Check sheet for the modelled part. Datum: model origin and axes. Units: mm. Face numbers are marked on the shaded views. A direction names the side the tool comes from. Coordinates: 2 decimals unless noted, no trailing zeros.
1. Set-up check for the marked faces 4, 5 and 6: record each of +Z, -Z, +X, -X, +Y, -Y from which the full face is reachable in a straight line by a thin tool's end or side.
2. Gauge pin test, flat ends, axial feed: pin 1 Ø1 at (x, y) = (-130.5, 9.5) entering from +Z; pin 2 Ø10.5 at (x, z) = (-103.5, 16) entering from +Y; pin 3 Ø6.5 at (y, z) = (4.5, 18) entering from -X; pin 4 Ø11 at (x, z) = (-158.2, 21.01) entering from -Y. Record the tip position at first contact, or that the pin passes through.
3. Thickness scan on line 1 (X direction, y = -4, z = 22); line 2 (X direction, y = 14.5, z = 20.5); line 3 (X direction, y = -10, z = 17.5). Record the ranges inside material, lowest first.
4. Draft check along X on the marked faces 1, 2 and 3. Enter one of: released by +X, released by -X, zero draft, split by the parting line, or undercut.
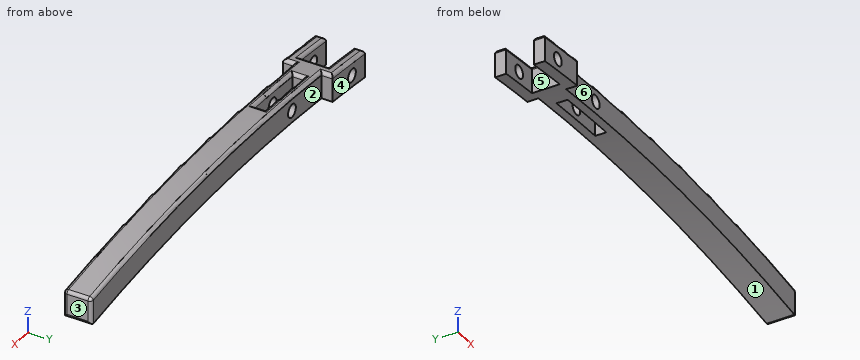
```python
from build123d import *

# Parameters (mm, degrees)
SKETCH011_W          = 60
SKETCH011_H          = 10
PAD005_DEPTH         = 40
POCKET002_DEPTH      = 35.001
POCKET002_DEPTH_BACK = 10.001
FILLET002_R          = 3
SKETCH013_R          = 6
POCKET003_DEPTH      = 35.001
POCKET003_DEPTH_BACK = 10.001


with BuildPart() as part:
    # Sketch011 → Pad005 (new body)
    with BuildSketch(Plane.XY):
        Polygon((-214, -12.5), (-214, 12.5), (-254, 12.5), (-254, 22.5), (-204, 22.5), (-204, 12.5), (152.4, 12.5), (152.4, -12.5), (-204, -12.5), (-204, -22.5), (-254, -22.5), (-254, -12.5), align=None)
        with Locations((-159, 0)):
            Rectangle(SKETCH011_W, SKETCH011_H, mode=Mode.SUBTRACT)
    extrude(amount=PAD005_DEPTH)

    # Sketch012 (on Face10 of Pad005) → Pocket002 (cut, two sides)
    with BuildSketch(Plane.XZ.offset(12.5)) as pocket002_sk:
        with BuildLine():
            ThreePointArc((152.4, 0), (-50.8, 13.99639), (-254, 0))
            Line((-254, 0), (152.4, 0))
        make_face()
        with BuildLine():
            ThreePointArc((152.4, 25), (-50.8, 38.764187), (-254, 25))
            Line((-254, 25), (-254, 40))
            Line((-254, 40), (152.4, 40))
            Line((152.4, 40), (152.4, 25))
        make_face()
    extrude(amount=-POCKET002_DEPTH, mode=Mode.SUBTRACT)
    extrude(pocket002_sk.sketch, amount=POCKET002_DEPTH_BACK, mode=Mode.SUBTRACT)

    # Fillet002
    fillet002_edges = [part.edges().sort_by_distance(p)[0] for p in [
        (152.4, 0, 0),
        (152.4, -12.5, 12.5),
        (152.4, 0, 25),
        (152.4, 12.5, 12.5),
        (-25.623265, -12.5, 38.553836),
        (-204, -17.5, 30.955836),
        (-229.02488, -22.5, 28.186792),
        (-254, -17.5, 25),
        (-234.016382, -12.5, 27.583774),
        (-214, 0, 29.900087),
        (-234.016382, 12.5, 27.583774),
        (-254, 17.5, 25),
        (-229.02488, 22.5, 28.186792),
        (-204, 17.5, 30.955836),
        (-25.623265, 12.5, 38.553836),
        (-189, 0, 32.41311),
        (-159.021563, -5, 34.872806),
        (-129, 0, 36.733601),
        (-159.021563, 5, 34.872806),
    ]]
    fillet(fillet002_edges, radius=FILLET002_R)

    # Sketch013 (on Face11 of Fillet002) → Pocket003 (cut, two sides)
    with BuildSketch(Plane.XZ.offset(12.5)) as pocket003_sk:
        with Locations((-158.200104, 21.012099)):
            Circle(SKETCH013_R)
        with Locations((-233.96661, 13.463589)):
            Circle(SKETCH013_R)
    extrude(amount=-POCKET003_DEPTH, mode=Mode.SUBTRACT)
    extrude(pocket003_sk.sketch, amount=POCKET003_DEPTH_BACK, mode=Mode.SUBTRACT)


solid = part.part
```
Data:
1. face 4: +Z, -Z, +X, -X, +Y
1. face 5: +Z, -Z, -X
1. face 6: +Z, -Z, +X, -Y
2. pin 1: stops at z = 36.68
2. pin 2: stops at y = 12.5
2. pin 3: stops at x = -214
2. pin 4: passes through
3. line 1: x = -214 to -189, -129 to 152.4
3. line 2: x = -254 to -204
3. line 3: x = -214 to -163.06, -153.34 to 152.36
4. face 1: undercut
4. face 2: zero draft
4. face 3: released by +X
